Can you work these out from the drawing? Everything is in mm from the part's minimum corner. Coordinates: 2 decimals unless noted, no trailing zeros. Loops run counter-clockwise (first coordinate to the right, second up) from the corner with the lowest first, then second, coordinate; pieces in that order, holes last. Notation, with made-up numbers: M -8.5,-18 L 37.5,-18 A19 cw 37.5,-5 Z; hole C 51.25,64 d7. An arc over 180 degrees is marked long. Use CSV: the item, a comma, the result in double quotes. Start each with the question number.
Q1. If we section it at D-D (x = 25.5): Please give me the cut outline in (y, z), and give its area (3 significant figures).
Q2. Please list where these lines run through material, in increasing order: probe 1 along Y at (x, z) = (15, 1.55); probe 2 along X at (y, z) = (11, 2.25); probe 3 along Z at (x, y) = (27, 6). Write a range as [from, to].
Q3. If we section it at A-A (y = 11): Please give me the cut outline in (x, z).
Q4. If we mould it in two halves opening along X, with no side actions, what happens to the marked faces 1, 2, 3 and 4? For each: +X half, -X half, draft (parallel to the pull), parting line (faces both ways), or undercut.
Q5. For pin 1 Ø2 at (x, y) = (19.5, 9) entering from +Z, with a flat end and sliding along its axis, tell me the tip position at first contact or that it passes through.
Q6. If we section it at B-B (x = 15): Please give me the cut outline in (y, z), and give its area (3 significant figures).
Q7. If we section it at C-C (z = 2.25): Please give me the cut outline in (x, y), and give its area (3 significant figures).
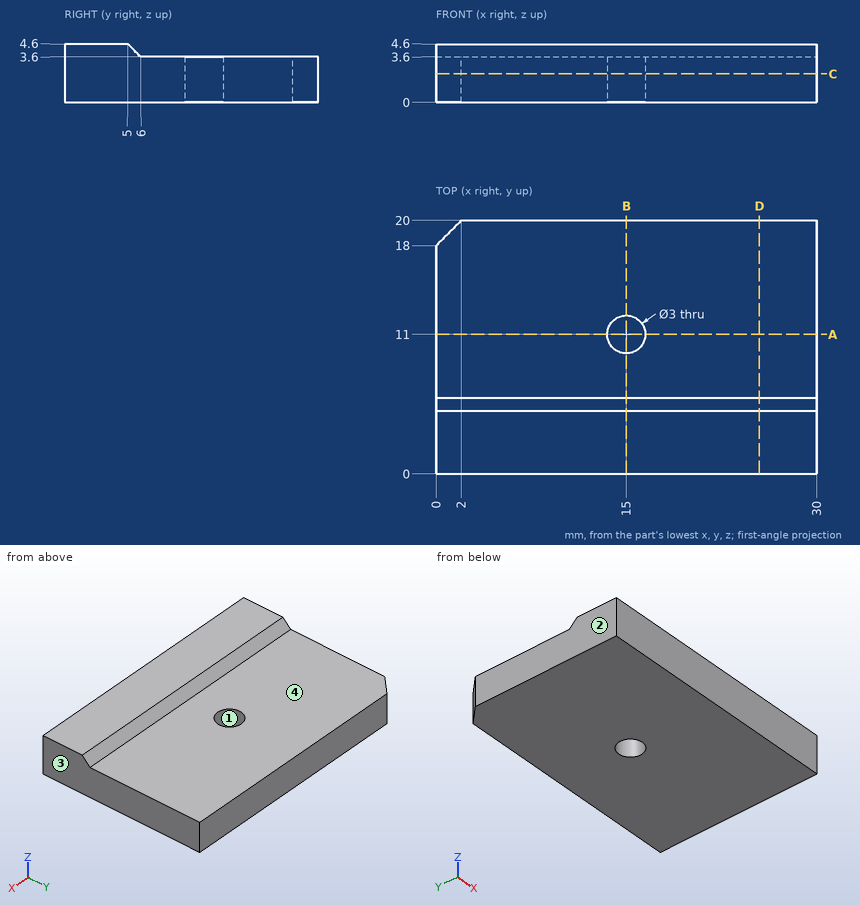
Results below:
1,outline,"M 0,0 L 20,0 L 20,3.6 L 6,3.6 L 5,4.6 L 0,4.6 Z"
1,area,"77.5 mm^2"
2,probe 1,"[0, 9.5], [12.5, 20]"
2,probe 2,"[0, 13.5], [16.5, 30]"
2,probe 3,"[0, 3.6]"
3,outline,"M 0,0 L 13.5,0 L 13.5,3.6 L 0,3.6 Z; M 16.5,0 L 30,0 L 30,3.6 L 16.5,3.6 Z"
4,face 1,"undercut"
4,face 2,"-X half"
4,face 3,"+X half"
4,face 4,"draft"
5,pin 1,"z = 3.6"
6,outline,"M 0,0 L 9.5,0 L 9.5,3.6 L 6,3.6 L 5,4.6 L 0,4.6 Z; M 12.5,0 L 20,0 L 20,3.6 L 12.5,3.6 Z"
6,area,"66.7 mm^2"
7,outline,"M 0,0 L 30,0 L 30,20 L 2,20 L 0,18 Z; hole C 15,11 d3"
7,area,"591 mm^2"
